```python
from build123d import *

# Parameters (mm, degrees)
F2_DEPTH = 30


# Not quite as in the source:
# - a feature of the source that left no trace in its solid (it failed there, or was rolled back) is left out


with BuildPart() as f2:
    # F1 (on Right) → F2 (new body)
    with BuildSketch(Plane.YZ):
        with BuildLine():
            Line((0, 25), (0, 0))
            ThreePointArc((0, 0), (3.4142135624, -1.4142135624), (2, 2))
            Line((2, 2), (2, 25))
            Line((2, 25), (0, 25))
        make_face()
        with BuildLine():
            ThreePointArc((3.01, 0), (2, -1.01), (0.99, 0))
            ThreePointArc((0.99, 0), (2, 1.01), (3.01, 0))
        make_face(mode=Mode.SUBTRACT)
    extrude(amount=F2_DEPTH)


solid = f2.part
```
Design review of the part built by this model. Coordinates are the model's own, in mm. A direction names the side the tool comes from. Give positions to 0.01 mm unless a question says otherwise; leave off trailing zeros. Loops run counter-clockwise (first coordinate to the right, second up) from the corner with the lowest first, then second, coordinate; pieces in that order, holes last. Notation, with made-up numbers: (28.5, 80.5) -> (86.5, 80.5) arc R26 cw to (86.5, 108.5) -> close; hole circle Ø7 at (-11, 52). An arc over 180 degrees is marked (long way). One line per item, written item: value.
Q1. For pin 1 Ø3 at (x, z) = (20, 20.5) entering from -Y; pin 2 Ø11.5 at (x, z) = (8.5, 13.5) entering from +Y, all flat-tipped, find the tip position at first contact; note any pin that passes through.
Numbers:
pin 1: stops at y = 0
pin 2: stops at y = 2
Q2. Machinability: for faces 5 (the flat face through (15, 2, 13)), 6 (the flat face through (30, 1, 12)), which of the approach directions +Z, -Z, +X, -X, +Y, -Y give a long, thin tool a straight path to every point of the face, cutting with its end or side? Answer none if there is none.
Numbers:
face 5: +Z, +X, -X, +Y
face 6: +Z, -Z, +X, +Y, -Y
Q3. For L1, parallel to Y at x = 20.5, z = 21.75; L2, parallel to Z at x = 14.5, y = 1.6; L3, parallel to Z at x = 21.5, y = 0.8, list the stretches that pass through material, from the lowest coordinate up.
Numbers:
L1: y = 0 to 2
L2: z = -1.96 to -0.93, 0.93 to 25
L3: z = -1.6 to 25
Q4. Draft analysis for pull direction Z (two halves, no side actions). For faces 1 (the flat face through (0, 1, 12)), 2 (the flat face through (15, 1, 25)), 3 (the cylindrical face through (14.79, 2.744, 0.683)), 4 (the cylindrical face through (14.79, 3.367, -1.46)), state which applies: pulls with the +Z half, pulls with the -Z half, needs draft (parallel to the pull), parting line crosses it, or undercut.
Numbers:
face 1: needs draft
face 2: pulls with the +Z half
face 3: undercut
face 4: parting line crosses it
Q5. We need section A-A on x = 4.75. Give the boundary of the cut face in (y, z), and give its area (3 significant figures).
Numbers:
outline: (0, 0) arc R2 ccw (long way) to (2, 2) -> (2, 25) -> (0, 25) -> close; hole circle Ø2.02 at (2, 0)
area: 56.2 mm^2
Q6. We need section B-B on z = 12.75. Give the boundary of the cut face in (x, y).
Numbers:
outline: (0, 0) -> (30, 0) -> (30, 2) -> (0, 2) -> close
